```python
from build123d import *

# Parameters (mm, degrees)
BOSS_EXTRUDE1_DEPTH = 9
SKETCH2_R           = 1
CUT_EXTRUDE1_DEPTH  = 2
FILLET1_R           = 1.27


with BuildPart() as part:
    # Sketch1 → Boss-Extrude1 (new body)
    with BuildSketch(Plane(origin=(0, 0, 0), x_dir=(1, 0, 0), z_dir=(0, 1, 0))):
        with BuildLine():
            Line((12.5, 0), (13.5, 0))
            Line((13.5, 0), (18.5, 0))
            Line((18.5, 0), (18.5, 1))
            Line((18.5, 1), (14.516, 1))
            ThreePointArc((14.516, 1), (13.79757951, 1.29757951), (13.5, 2.016))
            Line((13.5, 2.016), (13.5, 10.484))
            ThreePointArc((13.5, 10.484), (13.20242049, 11.20242049), (12.484, 11.5))
            Line((12.484, 11.5), (0.016, 11.5))
            ThreePointArc((0.016, 11.5), (-0.70242049, 11.20242049), (-1, 10.484))
            Line((-1, 10.484), (-1, 2.016))
            ThreePointArc((-1, 2.016), (-1.29757951, 1.29757951), (-2.016, 1))
            Line((-2.016, 1), (-6, 1))
            Line((-6, 1), (-6, 0))
            Line((-6, 0), (-0.999998, 0))
            Line((-0.999998, 0), (0, 0))
            Line((0, 0), (0, 9.484))
            ThreePointArc((0, 9.484), (0.29757951, 10.20242049), (1.016, 10.5))
            Line((1.016, 10.5), (11.484, 10.5))
            ThreePointArc((11.484, 10.5), (12.20242049, 10.20242049), (12.5, 9.484))
            Line((12.5, 9.484), (12.5, 0))
        make_face()
    extrude(amount=BOSS_EXTRUDE1_DEPTH)

    # Sketch2 → Cut-Extrude1 (cut, through all)
    with BuildSketch(Plane(origin=(0, 0, -1), x_dir=(-1, 0, 0), z_dir=(0, 0, -1))):
        with Locations((4, 2)):
            Circle(SKETCH2_R)
        with Locations((4, 7)):
            Circle(SKETCH2_R)
        with Locations((-16.5, 2)):
            Circle(SKETCH2_R)
        with Locations((-16.5, 7)):
            Circle(SKETCH2_R)
    extrude(amount=-CUT_EXTRUDE1_DEPTH, mode=Mode.SUBTRACT)

    # Fillet1
    fillet1_edges = [part.edges().sort_by_distance(p)[0] for p in [
        (-6, 0, -0.5),
        (18.5, 0, -0.5),
        (18.5, 9, -0.5),
        (-6, 9, -0.5),
    ]]
    fillet(fillet1_edges, radius=FILLET1_R)


solid = part.part
```
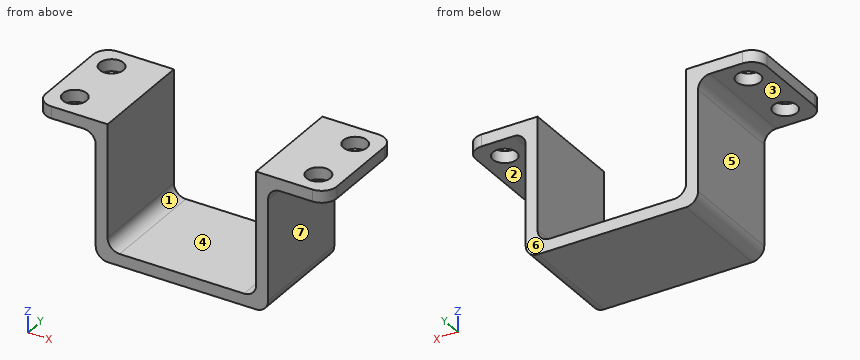
The listing builds one solid part. Answer for the finished solid, in the listing's coordinates (mm). Face numbers are marked on the shaded views. A direction names the side the tool comes from. Coordinates: 2 decimals unless noted, no trailing zeros. Loops run counter-clockwise (first coordinate to the right, second up) from the corner with the lowest first, then second, coordinate; pieces in that order, holes last. Notation, with made-up numbers: (-5, -29.75) - (29, -29.75) arc R22 cw to (29, -18.75) - close; hole circle Ø8 at (-22, -15). An arc over 180 degrees is marked (long way). Use a Markdown table: item, result. Add a question column.
1) The part is cut by section A-A, the plane y = 2. Give the vertices of the cut face in (x, z).
2) Find the intervals of material crossed by line 1 (Y direction, x = 16.5, z = -0.8); line 2 (X direction, y = 4.5, z = -6); line 3 (Z direction, x = 4, y = 5), in increasing order.
3) The part is cut by section C-C, the plane z = -5. Give the vertices of the cut face in (x, y), and give its area (3 significant figures).
4) Given pin 1 (2 mm diameter, centred on x = -3.5, y = 4.5, fed in from -Z); pin 2 (4 mm diameter, centred on x = 4, z = -9.5, fed in from -Y); pin 3 (1.5 mm diameter, centred on y = 6.5, z = -3, fed in from -X); pin 4 (2.5 mm diameter, centred on y = 2.5, z = -4.5, fed in from +X), each flat-ended and moving along its own axis, determine where each tip first touches the part or whether it passes through.
5) The part is cut by section B-B, the plane x = 16.5. Give the vertices of the cut face in (y, z), and give its area (3 significant figures).
6) The mould has two halves that part along X. Classify the marked faces 4, 5, 6 and 7: released by +X, released by -X, zero draft, split by the parting line, or undercut.
7) For the marked faces 1, 2 and 3, determine the directions among +Z, -Z, +X, -X, +Y, -Y from which every point of the face is accessible in a straight line to the end or side of a thin tool.
8) The part is cut by section D-D, the plane y = 4.5. Give the vertices of the cut face in (x, z).
Here are the results:
| question | item | result |
|---|---|---|
| 1 | outline | (-6, -1) - (-5, -1) - (-5, 0) - (-6, 0) - close; (-3, -1) - (-2.02, -1) arc R1.02 cw to (-1, -2.02) - (-1, -10.48) arc R1.02 ccw to (0.02, -11.5) - (12.48, -11.5) arc R1.02 ccw to (13.5, -10.48) - (13.5, -2.02) arc R1.02 cw to (14.52, -1) - (15.5, -1) - (15.5, 0) - (12.5, 0) - (12.5, -9.48) arc R1.02 cw to (11.48, -10.5) - (1.02, -10.5) arc R1.02 cw to (0, -9.48) - (0, 0) - (-3, 0) - close; (17.5, -1) - (18.5, -1) - (18.5, 0) - (17.5, 0) - close |
| 2 | line 1 | y = 0 to 1, 3 to 6, 8 to 9 |
| 2 | line 2 | x = -1 to 0, 12.5 to 13.5 |
| 2 | line 3 | z = -11.5 to -10.5 |
| 3 | outline | (-1, 0) - (0, 0) - (0, 9) - (-1, 9) - close; (12.5, 0) - (13.5, 0) - (13.5, 9) - (12.5, 9) - close |
| 3 | area | 18.0 mm^2 |
| 4 | pin 1 | stops at z = -1 |
| 4 | pin 2 | stops at y = 0 |
| 4 | pin 3 | stops at x = -1 |
| 4 | pin 4 | stops at x = 13.5 |
| 5 | outline | (0, -1) - (1, -1) - (1, 0) - (0, 0) - close; (3, -1) - (6, -1) - (6, 0) - (3, 0) - close; (8, -1) - (9, -1) - (9, 0) - (8, 0) - close |
| 5 | area | 5.00 mm^2 |
| 6 | face 4 | undercut |
| 6 | face 5 | released by -X |
| 6 | face 6 | zero draft |
| 6 | face 7 | released by +X |
| 7 | face 1 | +Z, +Y, -Y |
| 7 | face 2 | -Z, +X, +Y, -Y |
| 7 | face 3 | -Z, -X, +Y, -Y |
| 8 | outline | (-6, -1) - (-2.02, -1) arc R1.02 cw to (-1, -2.02) - (-1, -10.48) arc R1.02 ccw to (0.02, -11.5) - (12.48, -11.5) arc R1.02 ccw to (13.5, -10.48) - (13.5, -2.02) arc R1.02 cw to (14.52, -1) - (18.5, -1) - (18.5, 0) - (12.5, 0) - (12.5, -9.48) arc R1.02 cw to (11.48, -10.5) - (1.02, -10.5) arc R1.02 cw to (0, -9.48) - (0, 0) - (-6, 0) - close |
